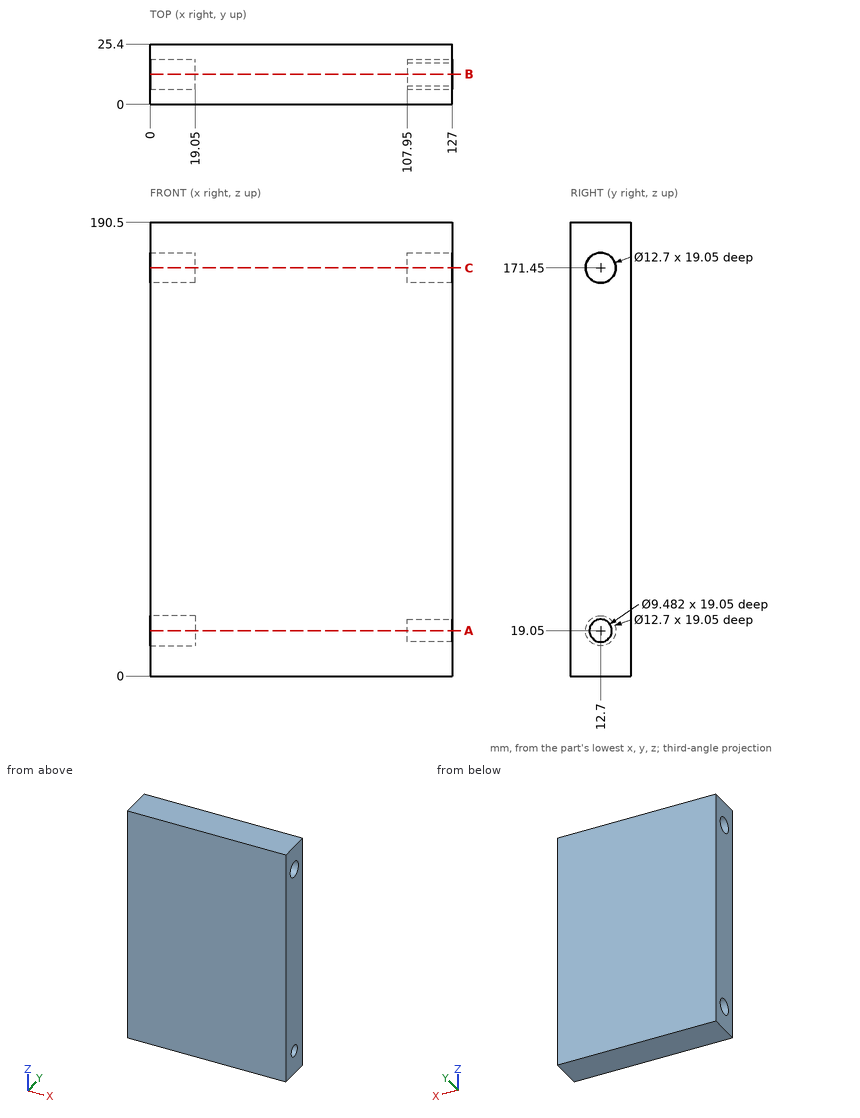
For this review, use the dimensioned drawing (mm, ordinates from the lowest corner) and the shaded views. Coordinates: 2 decimals unless noted, no trailing zeros. Order: outer loops, then holes, each group sorted by start corner. A loop starts at its lowest first (then second) coordinate and runs counter-clockwise, first axis right, second up. Notation, with made-up numbers: (60, 74) -> (73, 74) arc R25 cw to (73, 94) -> close; hole circle Ø9 at (-9.75, 65). An arc over 180 degrees is marked (long way). One line per item, written item: value. Start each with the question number.
Q1. Take a section at B-B, the plane y = 12.7. State the section outline as (x, z) points, then the cut area to 3 significant figures.
Q2. Take a section at A-A, the plane z = 19.05. State the section outline as (x, y) points.
Q3. Take a section at C-C, the plane z = 171.45. State the section outline as (x, y) points, then the cut area to 3 significant figures.
Q4. For probe 1 along Y at (x, z) = (122, 171.45); probe 2 along Y at (x, z) = (112, 19); probe 3 along X at (y, z) = (7.5, 22), list the stretches that pass through material, from the lowest coordinate up.
Q5. Insertion check: pin 1 Ø4 at (y, z) = (14, 19.5) entering from -X. The pin has a flat end and moves straight along its axis. Give the tip position at first contact, or say it passes through.
Values follow:
1. outline: (0, 0) -> (127, 0) -> (127, 14.31) -> (107.95, 14.31) -> (107.95, 23.79) -> (127, 23.79) -> (127, 165.1) -> (107.95, 165.1) -> (107.95, 177.8) -> (127, 177.8) -> (127, 190.5) -> (0, 190.5) -> (0, 177.8) -> (19.05, 177.8) -> (19.05, 165.1) -> (0, 165.1) -> (0, 25.4) -> (19.05, 25.4) -> (19.05, 12.7) -> (0, 12.7) -> close
1. area: 23,300 mm2
2. outline: (0, 0) -> (127, 0) -> (127, 7.96) -> (107.95, 7.96) -> (107.95, 17.44) -> (127, 17.44) -> (127, 25.4) -> (0, 25.4) -> (0, 19.05) -> (19.05, 19.05) -> (19.05, 6.35) -> (0, 6.35) -> close
3. outline: (0, 0) -> (127, 0) -> (127, 6.35) -> (107.95, 6.35) -> (107.95, 19.05) -> (127, 19.05) -> (127, 25.4) -> (0, 25.4) -> (0, 19.05) -> (19.05, 19.05) -> (19.05, 6.35) -> (0, 6.35) -> close
3. area: 2,740 mm2
4. probe 1: y = 0 to 6.35, 19.05 to 25.4
4. probe 2: y = 0 to 7.96, 17.44 to 25.4
4. probe 3: x = 19.05 to 127
5. pin 1: stops at x = 19.05
